Geometry: final body of the model. Coordinates: model frame, mm. A direction names the side the tool comes from. Give positions to 0.01 mm unless a question says otherwise; leave off trailing zeros. Order: outer loops, then holes, each group sorted by start corner. A loop starts at its lowest first (then second) coordinate and runs counter-clockwise, first axis right, second up. Notation, with made-up numbers: M -8.5,-12 L 43.5,-12 A11 ccw 43.5,1 Z; hole C -20.75,24 d5. An arc over 180 degrees is marked long. Use CSV: the item, a comma, the result in double quotes.
Autodesk Fusion 360 part; units mm, degrees
sketch "Sketch1" plane through (0, 0, 0) normal (0, 1, 0) x (1, 0, 0)
  arc A0 (-1.5, 2) -> (1.5, 2) centre (0, 0) ccw
  line L0 (1.5, 2) -> (-1.5, 2)
  circle A1 centre (0, 0) radius 3
  dimension "d2" = 3
  dimension "d3" = 2.5
  dimension "d4" = 6
extrude "Extrude1" add sketch "Sketch1" along normal blind 5
sketch "Sketch2" plane through (0, 5, 0) normal (0, 1, 0) x (-1, 0, 0)
  arc A0 (1.5, -2) -> (-1.5, -2) centre (0, 0) ccw
  line L0 (-1.5, -2) -> (1.5, -2)
  arc A1 (1.75, -3.5969) -> (1.75, 3.5969) centre (0, 0) ccw
  arc A2 (-1.75, 3.5969) -> (-1.75, -3.5969) centre (0, 0) ccw
  line L1 (-1.75, -3.5969) -> (1.75, -3.5969)
  line L2 (1.75, 3.5969) -> (-1.75, 3.5969)
  dimension "d7" = 3
  dimension "d8" = 2.5
  dimension "d9" = 4
  dimension "d10" = 4
  dimension "d11" = 3.5
  dimension "d12" = 3.5
extrude "Extrude2" add sketch "Sketch2" along normal blind 2.5
1. Reachability of faces 1 (the face through (4, 6, 0)), 2 (the face through (-3, 2, 0)) from +Z, -Z, +X, -X, +Y, -Y: full face, straight path, thin tool, end or side. Return the list, or none.
Answer:
face 1,"+X, +Y, -Y"
face 2,"-Y"
2. Section D-D, the plane y = 2.75. Return the cut outline in (x, z).
Answer:
outline,"C 0,0 d6; hole M -1.5,-2 L 1.5,-2 A2.5 ccw long Z"
3. Pull-direction query (X, two-part tool) for faces 3 (the face through (0, 6, 3.597)), 4 (the face through (0, 4, -2)), 5 (the face through (-4, 6, 0)); classes: +X half, -X half, draft (parallel to the pull), parting line (faces both ways), or undercut.
Answer:
face 3,"draft"
face 4,"undercut"
face 5,"-X half"
4. Section A-A, the plane x = 0. Return the cut outline in (y, z), plus the area to 3 significant figures.
Answer:
outline,"M 0,-3 L 5,-3 L 5,-3.6 L 7.5,-3.6 L 7.5,-2 L 0,-2 Z; M 0,2.5 L 7.5,2.5 L 7.5,3.6 L 5,3.6 L 5,3 L 0,3 Z"
area,"14.2 mm2"
5. Section B-B, the plane z = 0. Return the cut outline in (x, y).
Answer:
outline,"M -4,5 L -3,5 L -3,0 L -2.5,0 L -2.5,7.5 L -4,7.5 Z; M 2.5,0 L 3,0 L 3,5 L 4,5 L 4,7.5 L 2.5,7.5 Z"
6. Section C-C, the plane y = 6.75. Return the cut outline in (x, z).
Answer:
outline,"M -1.75,-3.6 L 1.75,-3.6 A4 ccw 1.75,3.6 L -1.75,3.6 A4 ccw Z; hole M -1.5,-2 L 1.5,-2 A2.5 ccw long Z"
7. Line query: line 1 (Z direction, x = 0, y = 2); line 2 (Y direction, x = 2.5, z = 2.5); line 3 (X direction, y = 6, z = 1.75). Output: solid intervals per line, ascending.
Answer:
line 1,"-3 to -2, 2.5 to 3"
line 2,"5 to 7.5"
line 3,"-3.6 to -1.79, 1.79 to 3.6"
8. Pin query (flat end, axial travel): pin 1 Ø3 at (x, z) = (-1.5, -1) entering from +Y; pin 2 Ø1.5 at (y, z) = (5.5, 1) entering from +X; pin 3 Ø0.9 at (x, y) = (0, 2) entering from +Z; pin 4 Ø3 at (x, y) = (2, 2.5) entering from -Z. Return the tip coordinate at first contact, or that it passes through.
Answer:
pin 1,"y = 7.5"
pin 2,"x = 3.99"
pin 3,"z = 3"
pin 4,"z = -2.96"
